from build123d import *

# Parameters (mm, degrees)
SKETCH1_W           = 150
SKETCH1_H           = 132.74
BOSS_EXTRUDE1_DEPTH = 5
SKETCH1_3_W         = 60
SKETCH1_3_H         = 6
SKETCH1_3_W_2       = 100
BOSS_EXTRUDE2_DEPTH = 15
FILLET1_R           = 1


with BuildPart() as part:
    # Sketch1 → Boss-Extrude1 (new body)
    with BuildSketch(Plane(origin=(0, 0, 0), x_dir=(1, 0, 0), z_dir=(0, 1, 0))):
        with Locations((0, -3.226)):
            Rectangle(SKETCH1_W, SKETCH1_H)
    extrude(amount=BOSS_EXTRUDE1_DEPTH)

    # Sketch1_3 → Boss-Extrude2 (add)
    with BuildSketch(Plane(origin=(0, 0, 0), x_dir=(1, 0, 0), z_dir=(0, 1, 0))):
        with Locations((-45, 60.144)):
            Rectangle(SKETCH1_3_W, SKETCH1_3_H)
        with Locations((-45, 40.096)):
            Rectangle(SKETCH1_3_W, SKETCH1_3_H)
        with Locations((45, 56.644)):
            Rectangle(SKETCH1_3_W, SKETCH1_3_H)
        with Locations((-45, 20.048)):
            Rectangle(SKETCH1_3_W, SKETCH1_3_H)
        with Locations((45, 36.596)):
            Rectangle(SKETCH1_3_W, SKETCH1_3_H)
        with Locations((-45, 0)):
            Rectangle(SKETCH1_3_W, SKETCH1_3_H)
        with Locations((45, 16.548)):
            Rectangle(SKETCH1_3_W, SKETCH1_3_H)
        with Locations((-45, -20.048)):
            Rectangle(SKETCH1_3_W, SKETCH1_3_H)
        with Locations((45, -3.5)):
            Rectangle(SKETCH1_3_W, SKETCH1_3_H)
        with Locations((-45, -40.096)):
            Rectangle(SKETCH1_3_W, SKETCH1_3_H)
        with Locations((45, -23.548)):
            Rectangle(SKETCH1_3_W, SKETCH1_3_H)
        with Locations((0, -66.596)):
            Rectangle(SKETCH1_3_W_2, SKETCH1_3_H)
        with Locations((45, -43.596)):
            Rectangle(SKETCH1_3_W, SKETCH1_3_H)
    extrude(amount=BOSS_EXTRUDE2_DEPTH)

    # Fillet1
    fillet1_edges = [part.edges().sort_by_distance(p)[0] for p in [
        (-15, 10, -3),
        (-75, 10, -3),
        (-75, 10, 3),
        (-15, 10, 3),
        (-15, 10, -23.048),
        (-75, 10, -23.048),
        (-75, 10, -17.048),
        (-15, 10, -17.048),
        (75, 2.5, -63.144),
        (75, 2.5, 69.596),
        (-75, 2.5, 69.596),
        (-75, 7.5, -63.144),
        (-15, 10, -43.096),
        (-75, 10, -43.096),
        (-75, 10, -37.096),
        (-15, 10, -37.096),
        (-75, 10, -57.144),
        (-15, 10, -57.144),
        (-15, 10, -63.144),
        (75, 10, -59.644),
        (15, 10, -59.644),
        (15, 10, -53.644),
        (75, 10, -53.644),
        (75, 10, -39.596),
        (15, 10, -39.596),
        (15, 10, -33.596),
        (75, 10, -33.596),
        (75, 10, -19.548),
        (15, 10, -19.548),
        (15, 10, -13.548),
        (75, 10, -13.548),
        (75, 10, 0.5),
        (15, 10, 0.5),
        (15, 10, 6.5),
        (75, 10, 6.5),
        (75, 10, 20.548),
        (15, 10, 20.548),
        (15, 10, 26.548),
        (75, 10, 26.548),
        (75, 10, 40.596),
        (15, 10, 40.596),
        (15, 10, 46.596),
        (75, 10, 46.596),
        (50, 10, 63.596),
        (-50, 10, 63.596),
        (-50, 10, 69.596),
        (50, 10, 69.596),
        (-15, 10, 37.096),
        (-75, 10, 37.096),
        (-75, 10, 43.096),
        (-15, 10, 43.096),
        (-15, 10, 17.048),
        (-75, 10, 17.048),
        (-75, 10, 23.048),
        (-15, 10, 23.048),
    ]]
    fillet(fillet1_edges, radius=FILLET1_R)


solid = part.part
Can you work these out from the model? Positions are in its coordinate system, mm. A direction names the side the tool comes from. Round coordinates to 2 decimals unless told otherwise and drop trailing zeros. Loops run counter-clockwise (first coordinate to the right, second up) from the corner with the lowest first, then second, coordinate; pieces in that order, holes last. Notation, with made-up numbers: (10, 49) - (57, 49) arc R22 cw to (57, 85) - close; hole circle Ø7 at (-25, -1.5). An arc over 180 degrees is marked (long way). Answer in a Markdown table with one row per item. Add a question column.
Q1. Which directions (+Z, -Z, +X, -X, +Y, -Y) give clear straight access to the entire face, cutting with the end or side of a thin tool? Please do faces 1 (the flat face through (-45, 10, -57.144)), 2 (the flat face through (45, 10, 46.596)), 3 (the flat face through (-50, 10, 67)), 4 (the flat face through (-15, 10, -20)).
Q2. I want a section at B-B on y = 8. Count the separate pieces of the cut face and the enclosed holes in it, and give its area (3 significant figures).
Q3. We'd pull the mould along X, two halves only. Please class faces 5 (the flat face through (75, 4, 4)), 6 (the flat face through (-15, 10, 20)), 7 (the flat face through (-45, 10, 37.096)), 8 (the flat face through (-75, 4, 4)): pulls with the +X half, pulls with the -X half, needs draft (parallel to the pull), parting line crosses it, or undercut.
Q4. I want a section at D-D on x = -38.5. List the corners of the cut face in (y, z) for me, and give its area (3 significant figures).
Q5. I need wall thicknesses on L1, parallel to Z at x = -64, y = 5.75; L2, parallel to Z at x = 61, y = 10.25; L3, parallel to Y at x = 56.5, z = 20. Which ranges of each line are inside material? Lowest first, please.
Q6. For pin 1 Ø1.2 at (y, z) = (12, -0.5) entering from +X; pin 2 Ø5 at (x, y) = (54.5, 8) entering from +Z; pin 3 Ø2 at (y, z) = (10.5, 66) entering from +X, each with a flat end and sliding along its axis, tell me the tip position at first contact or that it passes through.
Q7. I want a section at C-C on z = 60.5. List the corners of the cut face in (x, y) for me, and give its area (3 significant figures).
Q8. I want a section at A-A on x = 54. List the corners of the cut face in (y, z) for me, and give its area (3 significant figures).
A:
| question | item | result |
|---|---|---|
| 1 | face 1 | -X, +Y |
| 1 | face 2 | +X, -X, +Y |
| 1 | face 3 | +Z, -X, +Y |
| 1 | face 4 | -Z, +Y |
| 2 | separate pieces | 13 |
| 2 | enclosed holes | 0 |
| 2 | area | 4,910 mm^2 |
| 3 | face 5 | pulls with the +X half |
| 3 | face 6 | undercut |
| 3 | face 7 | needs draft |
| 3 | face 8 | pulls with the -X half |
| 4 | outline | (0, -63.14) - (15, -63.14) - (15, -57.14) - (5, -57.14) - (5, -43.1) - (15, -43.1) - (15, -37.1) - (5, -37.1) - (5, -23.05) - (15, -23.05) - (15, -17.05) - (5, -17.05) - (5, -3) - (15, -3) - (15, 3) - (5, 3) - (5, 17.05) - (15, 17.05) - (15, 23.05) - (5, 23.05) - (5, 37.1) - (15, 37.1) - (15, 43.1) - (5, 43.1) - (5, 63.6) - (15, 63.6) - (15, 69.6) - (0, 69.6) - close |
| 4 | area | 1,080 mm^2 |
| 5 | L1 | -63.14 to -57.14, -43.1 to -37.1, -23.05 to -17.05, -3 to 3, 17.05 to 23.05, 37.1 to 43.1 |
| 5 | L2 | -59.64 to -53.64, -39.6 to -33.6, -19.55 to -13.55, 0.5 to 6.5, 20.55 to 26.55, 40.6 to 46.6 |
| 5 | L3 | 0 to 5 |
| 6 | pin 1 | x = -15 |
| 6 | pin 2 | z = 46.6 |
| 6 | pin 3 | x = 50 |
| 7 | outline | (-75, 0) - (75, 0) - (75, 5) - (-75, 5) - close |
| 7 | area | 750 mm^2 |
| 8 | outline | (0, -63.14) - (5, -63.14) - (5, -59.64) - (15, -59.64) - (15, -53.64) - (5, -53.64) - (5, -39.6) - (15, -39.6) - (15, -33.6) - (5, -33.6) - (5, -19.55) - (15, -19.55) - (15, -13.55) - (5, -13.55) - (5, 0.5) - (15, 0.5) - (15, 6.5) - (5, 6.5) - (5, 20.55) - (15, 20.55) - (15, 26.55) - (5, 26.55) - (5, 40.6) - (15, 40.6) - (15, 46.6) - (5, 46.6) - (5, 69.6) - (0, 69.6) - close |
| 8 | area | 1,020 mm^2 |
